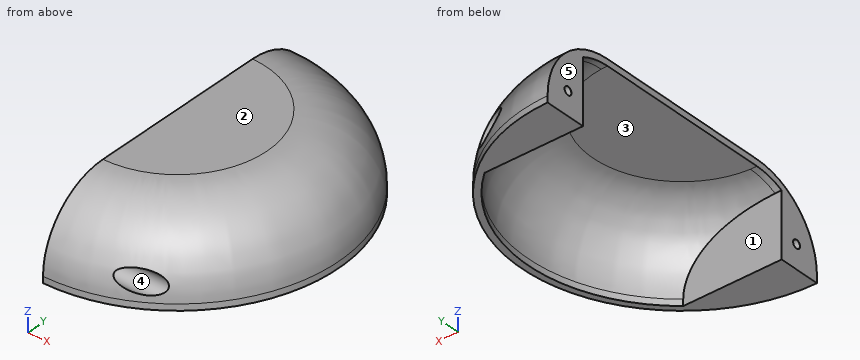
from build123d import *

# Parameters (mm, degrees)
SKETCH_1_R                     = 49.5
EXTRUDE_1_DEPTH                = 23.95
CUT_EXTRUDE_1_REACH            = 75.987
SKETCH_2_W                     = 51.856446696
SKETCH_2_H                     = 105.629558774
FILLET_1_R                     = 22
SHELL_1_T                      = -2
CUT_EXTRUDE_2_REACH            = 74.664
EXTRUDE_2_REACH                = 75.987
HOLE_WIZARD_M3_1_D             = 2.5
HOLE_WIZARD_M3_1_CSINK_D       = 2.55
HOLE_WIZARD_M3_1_CSINK_ANGLE   = 90
CUT_EXTRUDE_3_REACH            = 85.987
CUT_EXTRUDE_3_END_MAJOR_RADIUS = 27.5
CUT_EXTRUDE_3_END_MINOR_RADIUS = 22
CUT_EXTRUDE_START              = -10
SKETCH_9_R                     = 3.25


with BuildPart() as part:
    # 草图1 → 凸台-拉伸1 (new body)
    with BuildSketch(Plane.XY):
        Circle(SKETCH_1_R)
    extrude(amount=EXTRUDE_1_DEPTH)

    # 草图2 → 切除-拉伸1 (cut, up to next)
    with BuildSketch(Plane.XY, mode=Mode.PRIVATE) as cut_extrude_1_sk1:
        with Locations((-25.928223348, -1.331017626)):
            Rectangle(SKETCH_2_W, SKETCH_2_H)
    cut_extrude_1_tool1 = extrude(cut_extrude_1_sk1.sketch, amount=CUT_EXTRUDE_1_REACH, mode=Mode.PRIVATE) & part.part
    add(cut_extrude_1_tool1.solids().sort_by_distance((-25.928223, -1.331018, 0))[0], mode=Mode.SUBTRACT)

    # 圆角1
    fillet_1_edges = [part.edges().sort_by_distance(p)[0] for p in [
        (49.5, 0, 23.95),
    ]]
    fillet(fillet_1_edges, radius=FILLET_1_R)

    # 抽壳1
    shell_1_openings = [part.faces().sort_by_distance(p)[0] for p in [
        (21.008452488, 0, 0),
    ]]
    offset(amount=SHELL_1_T, openings=shell_1_openings)

    # 草图3 → 切除-拉伸2 (cut, up to next)
    with BuildSketch(Plane(origin=(2, 0, 0), x_dir=(0, 0, -1), z_dir=(1, 0, 0)), mode=Mode.PRIVATE) as cut_extrude_2_sk1:
        with BuildLine():
            Line((0, -47.457876059), (0, 47.457876059))
            Line((0, 47.457876059), (-1.95, 47.457876059))
            add(Edge.make_bspline(
                [(-1.95, 47.457876059), (-3.271867558, 47.457876059), (-4.580203295, 47.327986162), (-6.522470102, 46.938901335), (-7.160902253, 46.77755623), (-8.411173988, 46.395772827), (-9.637851686, 45.954297745), (-10.817777712, 45.394543369), (-11.973866888, 44.77448301), (-12.542496397, 44.432343138), (-14.177790511, 43.334814725), (-15.183450399, 42.505596807), (-16.567061926, 41.11769353), (-17.007634716, 40.630474323), (-17.843988232, 39.607544633), (-18.233424143, 39.079675999), (-19.318498452, 37.448564759), (-19.931677485, 36.298258611), (-20.683423408, 34.476900758), (-20.905979728, 33.851839293), (-21.284471808, 32.596856934), (-21.441928362, 31.963754853), (-21.820924381, 30.047967998), (-21.95, 28.748963189), (-21.95, 27.427176304)],
                knots=[0, 0, 0, 0, 0.125, 0.125, 0.1875, 0.1875, 0.25, 0.3125, 0.3125, 0.375, 0.375, 0.5, 0.5, 0.5625, 0.5625, 0.625, 0.625, 0.75, 0.75, 0.8125, 0.8125, 0.875, 0.875, 1, 1, 1, 1], degree=3))
            Line((-21.95, 27.427176304), (-21.95, -27.427176304))
            add(Edge.make_bspline(
                [(-21.95, -27.427176304), (-21.95, -28.748751501), (-21.820948006, -30.055931988), (-21.434879621, -31.995231967), (-21.273831263, -32.636531268), (-20.893390258, -33.888912081), (-20.453566277, -35.116841913), (-19.896522444, -36.29650639), (-19.279955682, -37.451662261), (-18.939789489, -38.019997246), (-17.843776455, -39.660921393), (-17.016258232, -40.668628413), (-15.633066823, -42.053808837), (-15.148182071, -42.494322146), (-14.129233176, -43.331552566), (-13.599488217, -43.724395897), (-11.969055187, -44.81417128), (-10.820320521, -45.429209656), (-9.003708201, -46.18303121), (-8.379162057, -46.406777614), (-7.12245463, -46.787996047), (-6.488637543, -46.946528678), (-4.571162151, -47.328045624), (-3.271637617, -47.457876059), (-1.95, -47.457876059)],
                knots=[0, 0, 0, 0, 0.125, 0.125, 0.1875, 0.1875, 0.25, 0.3125, 0.3125, 0.375, 0.375, 0.5, 0.5, 0.5625, 0.5625, 0.625, 0.625, 0.75, 0.75, 0.8125, 0.8125, 0.875, 0.875, 1, 1, 1, 1], degree=3))
            Line((-1.95, -47.457876059), (0, -47.457876059))
        make_face()
    cut_extrude_2_tool1 = extrude(cut_extrude_2_sk1.sketch, amount=-CUT_EXTRUDE_2_REACH, mode=Mode.PRIVATE) & part.part
    add(cut_extrude_2_tool1.solids().sort_by_distance((2, -4e-06, 10.389853))[0], mode=Mode.SUBTRACT)

    # 草图4 → 凸台-拉伸2 (add, up to next)
    with BuildSketch(Plane(origin=(0, 0, 0), x_dir=(-1, 0, 0), z_dir=(0, 0, -1)), mode=Mode.PRIVATE) as extrude_2_sk1:
        with BuildLine():
            Line((0, 36.5), (-30.397368307, 36.5))
            ThreePointArc((-30.397368307, 36.5), (-16.163229875, 44.665422868), (0, 47.5))
            Line((0, 47.5), (0, 36.5))
        make_face()
    extrude_2_tool1 = extrude(extrude_2_sk1.sketch, amount=-EXTRUDE_2_REACH, mode=Mode.PRIVATE) - part.part
    extrude_2 = extrude_2_tool1.solids().sort_by_distance((11.598273, 40.946819, 0))[0]
    add(extrude_2)

    # 镜向1: 凸台-拉伸2 mirrored; each copy of 凸台-拉伸2 runs up to whatever stops it at its own place
    mirror_1_before = part.part  # the part as the pattern finds it: every copy runs up to it
    mirror_1_extrude_2_long = extrude(extrude_2_sk1.sketch, amount=-EXTRUDE_2_REACH, mode=Mode.PRIVATE)
    mirror_1_extrude_2_tool1 = mirror_1_extrude_2_long.mirror(Plane.ZX) - mirror_1_before
    add(mirror_1_extrude_2_tool1.solids().sort_by_distance((11.598273, -40.946819, 0))[0])

    # M3 螺纹孔的螺纹孔钻头1 (through all)
    with Locations(Plane.ZY):
        with Locations((7.25, 42), (7.25, -42)):
            CounterSinkHole(HOLE_WIZARD_M3_1_D / 2, HOLE_WIZARD_M3_1_CSINK_D / 2, counter_sink_angle=HOLE_WIZARD_M3_1_CSINK_ANGLE)

    # 切除-拉伸3: up to this torus (the profile starts inside it)
    cut_extrude_3_end = Plane(origin=(0, 0, 1.95), z_dir=(0, 0, 1)) * Torus(CUT_EXTRUDE_3_END_MAJOR_RADIUS, CUT_EXTRUDE_3_END_MINOR_RADIUS, mode=Mode.PRIVATE)
    # 草图9 → 切除-拉伸3 (cut, up to the surface)
    with BuildSketch(Plane.ZY.offset(CUT_EXTRUDE_START), mode=Mode.PRIVATE) as cut_extrude_3_sk1:
        with Locations((7.25, 42)):
            Circle(SKETCH_9_R)
    cut_extrude_3_tool1 = extrude(cut_extrude_3_sk1.sketch, amount=-CUT_EXTRUDE_3_REACH, mode=Mode.PRIVATE) & cut_extrude_3_end
    add(cut_extrude_3_tool1.solids().sort_by_distance((10, 42, 7.25))[0], mode=Mode.SUBTRACT)
    # 草图9 → 切除-拉伸3 (cut, up to the surface)
    with BuildSketch(Plane.ZY.offset(CUT_EXTRUDE_START), mode=Mode.PRIVATE) as cut_extrude_3_sk2:
        with Locations((7.25, -42)):
            Circle(SKETCH_9_R)
    cut_extrude_3_tool2 = extrude(cut_extrude_3_sk2.sketch, amount=-CUT_EXTRUDE_3_REACH, mode=Mode.PRIVATE) & cut_extrude_3_end
    add(cut_extrude_3_tool2.solids().sort_by_distance((10, -42, 7.25))[0], mode=Mode.SUBTRACT)


solid = part.part
Read the model definition and answer for the solid it produces. Units are mm, in the model's axes. Face numbers are marked on the shaded views. A direction names the side the tool comes from. Give positions to 0.01 mm unless a question says otherwise; leave off trailing zeros. Write each loop counter-clockwise with the first axis right and the second up, starting at its lowest first coordinate (ties: lowest second). Pieces come first, ordered by that corner, then holes. Notation, with made-up numbers: M 19,26 L 64,26 A19 ccw 64,35 Z; hole C -31.5,-10.75 d5. An arc over 180 degrees is marked long. One line per item, written item: value. Start each with the question number.
(1) Find section B-B (z = 12.5). Determine the outline of the cut face in (x, y), plus the area to 3 significant figures.
(2) Find section A-A (z = 18.5). Determine the outline of the cut face in (x, y).
(3) A tool of negligible diameter and unlimited length cuts with its end or side. For the marked faces 3, 4 and 5, from which of +Z, -Z, +X, -X, +Y, -Y can it reach the whole face along a straight path? Write none if from no direction.
(4) Flat-ended cylindrical pins translate along their axes: pin 1 Ø10 at (y, z) = (-13, 15.5) entering from +X; pin 2 Ø10 at (y, z) = (3.5, 9) entering from +X; pin 3 Ø8 at (x, y) = (20.5, 3) entering from -Z. Find the tip coordinate at first contact, or state that the pin passes through.
(5) Determine the mould class of the marked faces 1 and 2 for opening direction Y: pulls with the +Y half, pulls with the -Y half, needs draft (parallel to the pull), parting line crosses it, or undercut.
(6) Find the intervals of material crossed by line 1 (Y direction, x = 6.5, z = 7.25); line 2 (Y direction, x = 19, z = 7.25); line 3 (Y direction, x = 4, z = 7.25), in increasing order.
Results below:
1. outline: M 0,-46.81 A46.81 ccw 0,46.81 L 0,36.5 L 25.44,36.5 A44.49 cw 25.44,-36.5 L 0,-36.5 Z
1. area: 608 mm^2
2. outline: M 0,-41.99 A41.99 ccw 0,41.99 L 0,36.5 L 12.95,36.5 A38.73 cw 12.95,-36.5 L 0,-36.5 Z
3. face 3: -Z, -X
3. face 4: +X
3. face 5: +Z, -Z, -X, +Y, -Y
4. pin 1: stops at x = 46.31
4. pin 2: stops at x = 49.34
4. pin 3: stops at z = 21.95
5. face 1: undercut
5. face 2: needs draft
6. line 1: y = -48.42 to -43.25, -40.75 to -36.5, 36.5 to 40.75, 43.25 to 48.42
6. line 2: y = -38.75 to -36.5, 36.5 to 38.75
6. line 3: y = -48.69 to -43.25, -40.75 to -36.5, 36.5 to 40.75, 43.25 to 48.69
